```python
from build123d import *

# Parameters (mm, degrees)
SKETCH_1_W             = 44
SKETCH_1_H             = 14.6
EXTRUDE_1_DEPTH        = 2
SKETCH_2_W             = 2.8
SKETCH_2_H             = 14.6
EXTRUDE_2_DEPTH        = 4
EXTRUDE_3_DEPTH        = 14.6
FILLET_1_R             = 1.2
FILLET_1_OF_MIRROR_1_R = 1.2


with BuildPart() as part:
    # 草图1 → 凸台-拉伸1 (new body)
    with BuildSketch(Plane.XY):
        Rectangle(SKETCH_1_W, SKETCH_1_H)
    extrude(amount=EXTRUDE_1_DEPTH)

    # 草图2 → 凸台-拉伸2 (add)
    with BuildSketch(Plane.XY.offset(2)):
        with Locations((20.6, 0)):
            Rectangle(SKETCH_2_W, SKETCH_2_H)
    extrude_2 = extrude(amount=EXTRUDE_2_DEPTH)

    # 草图3 → 凸台-拉伸3 (add)
    with BuildSketch(Plane.XZ.offset(7.3)):
        Polygon((22, 6), (20.4, 6), (20.4, 21.5), (24.9, 21.5), (24.9, 20.5), (22, 19), (22, 16.7), (23.2, 16.7), (23.2, 15.9), (22, 10), align=None)
    extrude_3 = extrude(amount=-EXTRUDE_3_DEPTH)

    # 圆角1
    fillet_1_edges = [part.edges().sort_by_distance(p)[0] for p in [
        (20.4, 0, 6),
    ]]
    fillet(fillet_1_edges, radius=FILLET_1_R - 0.0001)  # a hair under: the kernel refuses the full size

    # 镜向1: 凸台-拉伸2, 凸台-拉伸3 across plane
    add(extrude_2.mirror(Plane(origin=(0, 0, 0), x_dir=(0, 0, 1), z_dir=(1, 0, 0))))
    add(extrude_3.mirror(Plane(origin=(0, 0, 0), x_dir=(0, 0, 1), z_dir=(1, 0, 0))))

    # 圆角1 of 镜向1
    fillet_1_of_mirror_1_edges = [part.edges().sort_by_distance(p)[0] for p in [
        (-20.4, 0, 6),
    ]]
    fillet(fillet_1_of_mirror_1_edges, radius=FILLET_1_OF_MIRROR_1_R - 0.0001)  # a hair under: the kernel refuses the full size


solid = part.part
```
Work out the finished part from the listing and answer in its coordinate system (mm). A direction names the side the tool comes from. Coordinates: 2 decimals unless noted, no trailing zeros. Loops run counter-clockwise (first coordinate to the right, second up) from the corner with the lowest first, then second, coordinate; pieces in that order, holes last.
1) Section D-D (x = 15.5) is taken. Give the vertices of the cut face in (y, z), plus the area to 3 significant figures.
Results:
outline: (-7.3, 0) - (7.3, 0) - (7.3, 2) - (-7.3, 2) - close
area: 29.2 mm2
2) For a pull along X with two mould halves and no side action, classify faces 4 (the flat face through (-23, 0, 21.5)), 5 (the cylindrical face through (-20.058, 0.102, 6.361)), 6 (the flat face through (22, 0, 18)) as +X half, -X half, draft (parallel to the pull), parting line (faces both ways), or undercut.
Results:
face 4: draft
face 5: undercut
face 6: +X half
3) For faces 1 (the flat face through (23.47, -0.1, 19.76)), 2 (the flat face through (0, 0, 2)), 3 (the flat face through (-22, 0, 18)), determine the directions among +Z, -Z, +X, -X, +Y, -Y from which every point of the face is accessible in a straight line to the end or side of a thin tool.
Results:
face 1: +X, +Y, -Y
face 2: +Z, +Y, -Y
face 3: -X, +Y, -Y
4) Flat-ended cylindrical pins translate along their axes: pin 1 (2 mm diameter, centred on y = -2, z = 5, fed in from +X); pin 2 (0.6 mm diameter, centred on y = -0.5, z = 16.5, fed in from +X); pin 3 (2 mm diameter, centred on x = -9.5, y = -4, fed in from +Z). Find the tip coordinate at first contact, or state that the pin passes through.
Results:
pin 1: stops at x = 22
pin 2: stops at x = 23.2
pin 3: stops at z = 2
5) Section C-C (z = 4.25) is taken. Give the vertices of the cut face in (x, y).
Results:
outline: (-22, -7.3) - (-19.2, -7.3) - (-19.2, 7.3) - (-22, 7.3) - close; (19.2, -7.3) - (22, -7.3) - (22, 7.3) - (19.2, 7.3) - close
6) Consider probe 1 along X at (y, z) = (-4.5, 18); probe 2 along X at (y, z) = (4, 4.25); probe 3 along Z at (x, y) = (-11, 2.25). Determine where each line is inside the solid, lowest interval first.
Results:
probe 1: x = -22 to -20.4, 20.4 to 22
probe 2: x = -22 to -19.2, 19.2 to 22
probe 3: z = 0 to 2
7) Section A-A (z = 8.25) is taken. Give the vertices of the cut face in (x, y), plus the area to 3 significant figures.
Results:
outline: (-22, -7.3) - (-20.4, -7.3) - (-20.4, 7.3) - (-22, 7.3) - close; (20.4, -7.3) - (22, -7.3) - (22, 7.3) - (20.4, 7.3) - close
area: 46.7 mm2
